Input: part model. Units: mm. Frame: model coordinates. A direction names the side the tool comes from. Round coordinates to 2 decimals unless told otherwise and drop trailing zeros. Order: outer loops, then holes, each group sorted by start corner. A loop starts at its lowest first (then second) coordinate and runs counter-clockwise, first axis right, second up.
Item 1: Cut plane D-D on y = 28. Output: boundary loops of the cut face in (x, z), then the cut area to 3 significant figures.
Item 2: Reachability of faces 5 (the flat face through (-1, 7, -2.5)), 6 (the flat face through (-1, 40, -43.5)) from +Z, -Z, +X, -X, +Y, -Y: full face, straight path, thin tool, end or side. Return the list, or none.
Item 3: Cut plane B-B on x = 2.75. Output: boundary loops of the cut face in (y, z), then the cut area to 3 significant figures.
Item 4: Cut plane C-C on z = -15. Output: boundary loops of the cut face in (x, y).
Item 5: Line query: L1, parallel to Z at x = 2, y = -1.5; L2, parallel to Y at x = -7.75, z = -16; L3, parallel to Y at x = 1, z = -11.5. Output: solid intervals per line, ascending.
Item 6: First-contact query: pin 1 (4 mm diameter, centred on x = -2, z = -20, fed in from -Y); pin 2 (3.5 mm diameter, centred on x = -0.5, y = -31.5, fed in from -Z); pin 3 (4 mm diameter, centred on x = 2.5, y = 20.5, fed in from -Z); pin 4 (4 mm diameter, centred on y = -22.5, z = -5.5, fed in from -X). Flat tips, straight axial feed; report the tip coordinate or a pass-through.
Item 7: Cut plane A-A on z = -36.5. Output: boundary loops of the cut face in (x, y), then the cut area to 3 significant figures.
Item 8: Mould query, pull axis Y, two halves, no side actions, for faces 1 (the flat face through (-1, -36.93, -5)), 2 (the flat face through (-1, -31, -12.5)), 3 (the flat face through (-1, 38.07, -23)), 4 (the flat face through (-1, -24.93, -7)). Classes: released by +Y, released by -Y, zero draft, split by the parting line, or undercut.
```python
from build123d import *

# Parameters (mm, degrees)
F0_W     = 20
F0_H     = 63
F1_DEPTH = 2.5
F2_W     = 20
F2_H     = 15
F3_DEPTH = 12
F4_W     = 20
F4_H     = 46
F5_DEPTH = 3
F6_R     = 1.5
F7_DEPTH = 25


with BuildPart() as f1:
    # F0 (on Top) → F1 (new body, symmetric)
    with BuildSketch(Plane.XY):
        with Locations((-1.321708, 6.569935)):
            Rectangle(F0_W, F0_H)
    extrude(amount=F1_DEPTH, both=True)

    # F2 (on face) → F3 (join)
    with BuildSketch(Plane.XZ.offset(24.930065)):
        with Locations((-1.321708, -5)):
            Rectangle(F2_W, F2_H)
    extrude(amount=F3_DEPTH)

    # F4 (on face) → F5 (join)
    with BuildSketch(Plane(origin=(0, 38.069935, 0), x_dir=(-1, 0, 0), z_dir=(0, 1, 0))):
        with Locations((1.321708, -20.5)):
            Rectangle(F4_W, F4_H)
    extrude(amount=F5_DEPTH)

    # F6 (on face) → F7 (cut)
    with BuildSketch(Plane(origin=(0, 41.069935, 0), x_dir=(-1, 0, 0), z_dir=(0, 1, 0))):
        with Locations((5.321708, -36.5)):
            Circle(F6_R)
    extrude(amount=-F7_DEPTH, mode=Mode.SUBTRACT)


solid = f1.part
```
From the geometry:
1. outline: (-11.32, -2.5) - (8.68, -2.5) - (8.68, 2.5) - (-11.32, 2.5) - close
1. area: 100 mm2
2. face 5: -Z, +X, -X
2. face 6: -Z, +X, -X, +Y, -Y
3. outline: (-36.93, -12.5) - (-24.93, -12.5) - (-24.93, -2.5) - (38.07, -2.5) - (38.07, -43.5) - (41.07, -43.5) - (41.07, 2.5) - (-36.93, 2.5) - close
3. area: 633 mm2
4. outline: (-11.32, 38.07) - (8.68, 38.07) - (8.68, 41.07) - (-11.32, 41.07) - close
5. L1: z = -2.5 to 2.5
5. L2: y = 38.07 to 41.07
5. L3: y = -36.93 to -24.93, 38.07 to 41.07
6. pin 1: stops at y = 38.07
6. pin 2: stops at z = -12.5
6. pin 3: stops at z = -2.5
6. pin 4: passes through
7. outline: (-11.32, 38.07) - (-6.82, 38.07) - (-6.82, 41.07) - (-11.32, 41.07) - close; (-3.82, 38.07) - (8.68, 38.07) - (8.68, 41.07) - (-3.82, 41.07) - close
7. area: 51.0 mm2
8. face 1: released by -Y
8. face 2: zero draft
8. face 3: undercut
8. face 4: undercut
